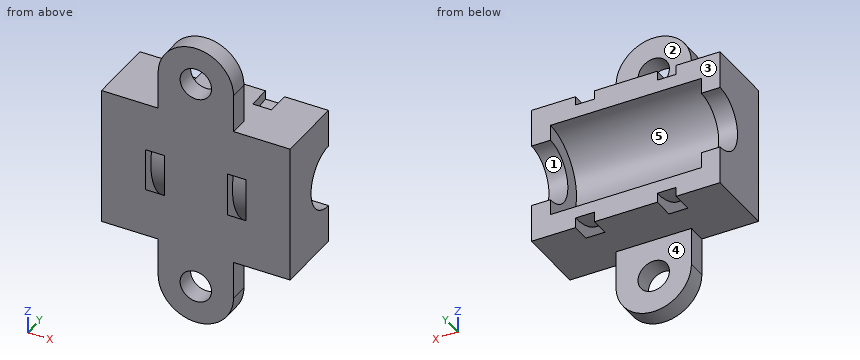
```python
from build123d import *

# Parameters (mm, degrees)
CROQUIS1_W              = 30
CROQUIS1_H              = 22
SALIENTE_EXTRUIR1_DEPTH = 11
CROQUIS2_R              = 2.5
SALIENTE_EXTRUIR2_DEPTH = 3
CROQUIS3_R              = 5
CORTAR_EXTRUIR1_DEPTH   = 31
CROQUIS4_R              = 11.5
CROQUIS4_R_2            = 9.5
CORTAR_EXTRUIR13_DEPTH  = 3
CROQUIS6_R              = 11.5
CROQUIS6_R_2            = 9.5
CORTAR_EXTRUIR14_DEPTH  = 3
CROQUIS7_R              = 7.5
CORTAR_EXTRUIR15_DEPTH  = 24


with BuildPart() as part:
    # Croquis1 → Saliente-Extruir1 (new body)
    with BuildSketch(Plane(origin=(0, 0, 0), x_dir=(1, 0, 0), z_dir=(0, 1, 0))):
        with Locations((15, 11)):
            Rectangle(CROQUIS1_W, CROQUIS1_H)
    extrude(amount=SALIENTE_EXTRUIR1_DEPTH)

    # Croquis2 → Saliente-Extruir2 (add)
    with BuildSketch(Plane.XZ):
        with BuildLine():
            Line((21, 6), (21, 0))
            Line((21, 0), (9, 0))
            Line((9, 0), (9, 6))
            ThreePointArc((9, 6), (15, 12), (21, 6))
        make_face()
        with Locations((15, 6)):
            Circle(CROQUIS2_R, mode=Mode.SUBTRACT)
        with BuildLine():
            Line((9, -22), (9, -28))
            ThreePointArc((9, -28), (15, -34), (21, -28))
            Line((21, -28), (21, -22))
            Line((21, -22), (9, -22))
        make_face()
        with Locations((15, -28)):
            Circle(CROQUIS2_R, mode=Mode.SUBTRACT)
    extrude(amount=-SALIENTE_EXTRUIR2_DEPTH)

    # Croquis3 → Cortar-Extruir1 (cut, through all)
    with BuildSketch(Plane.ZY):
        with Locations((-11, 11)):
            Circle(CROQUIS3_R)
    extrude(amount=-CORTAR_EXTRUIR1_DEPTH, mode=Mode.SUBTRACT)

    # Croquis4 → Cortar-Extruir13 (cut)
    with BuildSketch(Plane.ZY.offset(-10)):
        with Locations((-11, 11)):
            Circle(CROQUIS4_R)
        with Locations((-11, 11)):
            Circle(CROQUIS4_R_2, mode=Mode.SUBTRACT)
    extrude(amount=CORTAR_EXTRUIR13_DEPTH, mode=Mode.SUBTRACT)

    # Croquis6 → Cortar-Extruir14 (cut)
    with BuildSketch(Plane(origin=(20, 0, 0), x_dir=(0, 0, -1), z_dir=(1, 0, 0))):
        with Locations((10.887185848, 10.972715561)):
            Circle(CROQUIS6_R)
        with Locations((10.887185848, 10.972715561)):
            Circle(CROQUIS6_R_2, mode=Mode.SUBTRACT)
    extrude(amount=CORTAR_EXTRUIR14_DEPTH, mode=Mode.SUBTRACT)

    # Croquis7 → Cortar-Extruir15 (cut)
    with BuildSketch(Plane.ZY.offset(-3)):
        with Locations((-11, 11)):
            Circle(CROQUIS7_R)
    extrude(amount=-CORTAR_EXTRUIR15_DEPTH, mode=Mode.SUBTRACT)


solid = part.part
```
CAD build for the part. Positions are in the model's coordinates, mm. Face numbers are marked on the shaded views. A direction names the side the tool comes from. Coordinates: 2 decimals unless noted, no trailing zeros. Write each loop counter-clockwise with the first axis right and the second up, starting at its lowest first coordinate (ties: lowest second). Pieces come first, ordered by that corner, then holes.
(1) Cut at D-D, the plane z = -2.5. List the corners of the cut face in (x, y), and give its area (3 significant figures).
(2) 3-axis set-ups, long thin cutter, end or side, ignore diameter. For the marked faces 3, 4 and 5: which of +Z, -Z, +X, -X, +Y, -Y reach the whole face in a straight line?
(3) Cut at B-B, the plane z = -27. List the corners of the cut face in (x, y).
(4) Cut at C-C, the plane x = 6.25. List the corners of the cut face in (y, z).
(5) Two-plate mould, pull along Z, no slides. Class the marked faces 1 and 2: +Z half, -Z half, draft (parallel to the pull), parting line (faces both ways), or undercut.
(6) Flat gauge pins, fed straight in: pin 1 (4 mm diameter, centred on x = 15, z = -28, fed in from +Y); pin 2 (1.5 mm diameter, centred on x = 18, y = 1.5, fed in from +Z); pin 3 (0.9 mm diameter, centred on y = 1.5, z = -25.5, fed in from +X); pin 4 (5.5 mm diameter, centred on x = 16, y = 3.5, fed in from +Z). Where does each tip first touch, or does it go through?
(7) Cut at A-A, the plane x = 15. List the corners of the cut face in (y, z).
(8) Drill centre lines: probe 1 along X at (y, z) = (8.25, -20.5); probe 2 along Z at (x, y) = (15, 2.3); probe 3 along Z at (x, y) = (15.5, 1). Where is each one in solid material? Low to high.
Geometry says:
1. outline: (0, 0) - (30, 0) - (30, 11) - (0, 11) - close; hole (7, 3.25) - (10, 3.25) - (10, 6.76) - (7, 6.76) - close; hole (20, 3.1) - (23, 3.1) - (23, 6.51) - (20, 6.51) - close
1. area: 309 mm2
2. face 3: +Z, -Z, +X, -X, +Y
2. face 4: -Z, +X, -X, +Y
2. face 5: +Y
3. outline: (9, 0) - (12.71, 0) - (12.71, 3) - (9, 3) - close; (17.29, 0) - (21, 0) - (21, 3) - (17.29, 3) - close
4. outline: (0, -22) - (11, -22) - (11, -18.5) arc R7.5 cw to (11, -3.5) - (11, 0) - (0, 0) - close
5. face 1: undercut
5. face 2: draft
6. pin 1: passes through
6. pin 2: stops at z = 11.56
6. pin 3: stops at x = 21
6. pin 4: stops at z = 12
7. outline: (0, -34) - (3, -34) - (3, -30.5) - (0, -30.5) - close; (0, -25.5) - (3, -25.5) - (3, -22) - (11, -22) - (11, -18.5) arc R7.5 cw to (11, -3.5) - (11, 0) - (3, 0) - (3, 3.5) - (0, 3.5) - close; (0, 8.5) - (3, 8.5) - (3, 12) - (0, 12) - close
8. probe 1: x = 0 to 7, 10 to 20, 23 to 30
8. probe 2: z = -34 to -30.5, -25.5 to 3.5, 8.5 to 12
8. probe 3: z = -33.98 to -30.45, -25.55 to 3.55, 8.45 to 11.98
